Design review of the part built by this model. Coordinates are the model's own, in mm. Coordinates: 2 decimals unless noted, no trailing zeros. Loops run counter-clockwise (first coordinate to the right, second up) from the corner with the lowest first, then second, coordinate; pieces in that order, holes last. Notation, with made-up numbers: (-9, 27) -> (0, 27) arc R18 cw to (0, 32) -> close; hole circle Ø4 at (-35.5, 41). An arc over 180 degrees is marked (long way). Use one line per item in the form item = value. Start each with the question number.
1. Consider section A-A (z = 17.5). State the section outline as (x, y) points, then the cut area to 3 significant figures.
2. Consider section B-B (x = -33). State the section outline as (y, z) points.
3. For pin 1 (1.3 mm diameter, centred on y = 1, z = -22.5, fed in from -X); pin 2 (1.3 mm diameter, centred on y = 1.5, z = 18, fed in from +X), all flat-tipped, find the tip position at first contact; note any pin that passes through.
4. Wall thickness on line 1 (X direction, y = 0.9, z = 3.5); line 2 (Z direction, x = 44, y = 1.55): over which ranges is each line inside the solid? List them lowest first. Write a range as from..to.
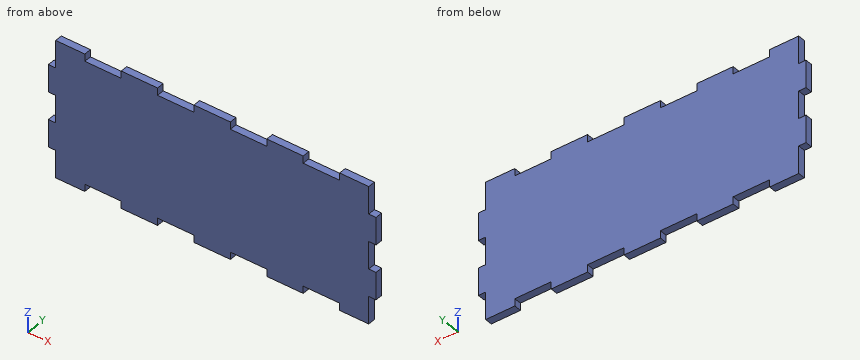
from build123d import *

# Parameters (mm, degrees)
SKETCH1_W           = 114.3
SKETCH1_H           = 48.006
BOSS_EXTRUDE1_DEPTH = 2.54
CUT_EXTRUDE2_REACH  = 64.038
SKETCH2_W           = 2.54
SKETCH2_H           = 9.6012
SKETCH2_W_2         = 12.7
SKETCH2_H_2         = 2.54


with BuildPart() as part:
    # Sketch1 → Boss-Extrude1 (new body)
    with BuildSketch(Plane(origin=(0, 0, 0), x_dir=(1, 0, 0), z_dir=(0, 1, 0))):
        Rectangle(SKETCH1_W, SKETCH1_H)
    extrude(amount=BOSS_EXTRUDE1_DEPTH)

    # Sketch2 → Cut-Extrude2 (cut, up to next)
    with BuildSketch(Plane(origin=(0, 2.54, 0), x_dir=(1, 0, 0), z_dir=(0, 1, 0)), mode=Mode.PRIVATE) as cut_extrude2_sk1:
        with Locations((-55.88, 19.2024)):
            Rectangle(SKETCH2_W, SKETCH2_H)
    cut_extrude2_tool1 = extrude(cut_extrude2_sk1.sketch, amount=-CUT_EXTRUDE2_REACH, mode=Mode.PRIVATE) & part.part
    # Sketch2 → Cut-Extrude2 (cut, up to next)
    with BuildSketch(Plane(origin=(0, 2.54, 0), x_dir=(1, 0, 0), z_dir=(0, 1, 0)), mode=Mode.PRIVATE) as cut_extrude2_sk2:
        with Locations((-38.1, 22.733)):
            Rectangle(SKETCH2_W_2, SKETCH2_H_2)
    cut_extrude2_tool2 = extrude(cut_extrude2_sk2.sketch, amount=-CUT_EXTRUDE2_REACH, mode=Mode.PRIVATE) & part.part
    # Sketch2 → Cut-Extrude2 (cut, up to next)
    with BuildSketch(Plane(origin=(0, 2.54, 0), x_dir=(1, 0, 0), z_dir=(0, 1, 0)), mode=Mode.PRIVATE) as cut_extrude2_sk3:
        with Locations((-12.7, 22.733)):
            Rectangle(SKETCH2_W_2, SKETCH2_H_2)
    cut_extrude2_tool3 = extrude(cut_extrude2_sk3.sketch, amount=-CUT_EXTRUDE2_REACH, mode=Mode.PRIVATE) & part.part
    # Sketch2 → Cut-Extrude2 (cut, up to next)
    with BuildSketch(Plane(origin=(0, 2.54, 0), x_dir=(1, 0, 0), z_dir=(0, 1, 0)), mode=Mode.PRIVATE) as cut_extrude2_sk4:
        with Locations((12.7, 22.733)):
            Rectangle(SKETCH2_W_2, SKETCH2_H_2)
    cut_extrude2_tool4 = extrude(cut_extrude2_sk4.sketch, amount=-CUT_EXTRUDE2_REACH, mode=Mode.PRIVATE) & part.part
    # Sketch2 → Cut-Extrude2 (cut, up to next)
    with BuildSketch(Plane(origin=(0, 2.54, 0), x_dir=(1, 0, 0), z_dir=(0, 1, 0)), mode=Mode.PRIVATE) as cut_extrude2_sk5:
        with Locations((38.1, 22.733)):
            Rectangle(SKETCH2_W_2, SKETCH2_H_2)
    cut_extrude2_tool5 = extrude(cut_extrude2_sk5.sketch, amount=-CUT_EXTRUDE2_REACH, mode=Mode.PRIVATE) & part.part
    # Sketch2 → Cut-Extrude2 (cut, up to next)
    with BuildSketch(Plane(origin=(0, 2.54, 0), x_dir=(1, 0, 0), z_dir=(0, 1, 0)), mode=Mode.PRIVATE) as cut_extrude2_sk6:
        with Locations((55.88, 19.2024)):
            Rectangle(SKETCH2_W, SKETCH2_H)
    cut_extrude2_tool6 = extrude(cut_extrude2_sk6.sketch, amount=-CUT_EXTRUDE2_REACH, mode=Mode.PRIVATE) & part.part
    # Sketch2 → Cut-Extrude2 (cut, up to next)
    with BuildSketch(Plane(origin=(0, 2.54, 0), x_dir=(1, 0, 0), z_dir=(0, 1, 0)), mode=Mode.PRIVATE) as cut_extrude2_sk7:
        with Locations((55.88, 0)):
            Rectangle(SKETCH2_W, SKETCH2_H)
    cut_extrude2_tool7 = extrude(cut_extrude2_sk7.sketch, amount=-CUT_EXTRUDE2_REACH, mode=Mode.PRIVATE) & part.part
    # Sketch2 → Cut-Extrude2 (cut, up to next)
    with BuildSketch(Plane(origin=(0, 2.54, 0), x_dir=(1, 0, 0), z_dir=(0, 1, 0)), mode=Mode.PRIVATE) as cut_extrude2_sk8:
        with Locations((55.88, -19.2024)):
            Rectangle(SKETCH2_W, SKETCH2_H)
    cut_extrude2_tool8 = extrude(cut_extrude2_sk8.sketch, amount=-CUT_EXTRUDE2_REACH, mode=Mode.PRIVATE) & part.part
    # Sketch2 → Cut-Extrude2 (cut, up to next)
    with BuildSketch(Plane(origin=(0, 2.54, 0), x_dir=(1, 0, 0), z_dir=(0, 1, 0)), mode=Mode.PRIVATE) as cut_extrude2_sk9:
        with Locations((38.1, -22.733)):
            Rectangle(SKETCH2_W_2, SKETCH2_H_2)
    cut_extrude2_tool9 = extrude(cut_extrude2_sk9.sketch, amount=-CUT_EXTRUDE2_REACH, mode=Mode.PRIVATE) & part.part
    # Sketch2 → Cut-Extrude2 (cut, up to next)
    with BuildSketch(Plane(origin=(0, 2.54, 0), x_dir=(1, 0, 0), z_dir=(0, 1, 0)), mode=Mode.PRIVATE) as cut_extrude2_sk10:
        with Locations((12.7, -22.733)):
            Rectangle(SKETCH2_W_2, SKETCH2_H_2)
    cut_extrude2_tool10 = extrude(cut_extrude2_sk10.sketch, amount=-CUT_EXTRUDE2_REACH, mode=Mode.PRIVATE) & part.part
    # Sketch2 → Cut-Extrude2 (cut, up to next)
    with BuildSketch(Plane(origin=(0, 2.54, 0), x_dir=(1, 0, 0), z_dir=(0, 1, 0)), mode=Mode.PRIVATE) as cut_extrude2_sk11:
        with Locations((-12.7, -22.733)):
            Rectangle(SKETCH2_W_2, SKETCH2_H_2)
    cut_extrude2_tool11 = extrude(cut_extrude2_sk11.sketch, amount=-CUT_EXTRUDE2_REACH, mode=Mode.PRIVATE) & part.part
    # Sketch2 → Cut-Extrude2 (cut, up to next)
    with BuildSketch(Plane(origin=(0, 2.54, 0), x_dir=(1, 0, 0), z_dir=(0, 1, 0)), mode=Mode.PRIVATE) as cut_extrude2_sk12:
        with Locations((-38.1, -22.733)):
            Rectangle(SKETCH2_W_2, SKETCH2_H_2)
    cut_extrude2_tool12 = extrude(cut_extrude2_sk12.sketch, amount=-CUT_EXTRUDE2_REACH, mode=Mode.PRIVATE) & part.part
    # Sketch2 → Cut-Extrude2 (cut, up to next)
    with BuildSketch(Plane(origin=(0, 2.54, 0), x_dir=(1, 0, 0), z_dir=(0, 1, 0)), mode=Mode.PRIVATE) as cut_extrude2_sk13:
        with Locations((-55.88, -19.2024)):
            Rectangle(SKETCH2_W, SKETCH2_H)
    cut_extrude2_tool13 = extrude(cut_extrude2_sk13.sketch, amount=-CUT_EXTRUDE2_REACH, mode=Mode.PRIVATE) & part.part
    # Sketch2 → Cut-Extrude2 (cut, up to next)
    with BuildSketch(Plane(origin=(0, 2.54, 0), x_dir=(1, 0, 0), z_dir=(0, 1, 0)), mode=Mode.PRIVATE) as cut_extrude2_sk14:
        with Locations((-55.88, 0)):
            Rectangle(SKETCH2_W, SKETCH2_H)
    cut_extrude2_tool14 = extrude(cut_extrude2_sk14.sketch, amount=-CUT_EXTRUDE2_REACH, mode=Mode.PRIVATE) & part.part
    add(cut_extrude2_tool1.solids().sort_by_distance((-55.88, 2.54, -19.2024))[0], mode=Mode.SUBTRACT)
    add(cut_extrude2_tool2.solids().sort_by_distance((-38.1, 2.54, -22.733))[0], mode=Mode.SUBTRACT)
    add(cut_extrude2_tool3.solids().sort_by_distance((-12.7, 2.54, -22.733))[0], mode=Mode.SUBTRACT)
    add(cut_extrude2_tool4.solids().sort_by_distance((12.7, 2.54, -22.733))[0], mode=Mode.SUBTRACT)
    add(cut_extrude2_tool5.solids().sort_by_distance((38.1, 2.54, -22.733))[0], mode=Mode.SUBTRACT)
    add(cut_extrude2_tool6.solids().sort_by_distance((55.88, 2.54, -19.2024))[0], mode=Mode.SUBTRACT)
    add(cut_extrude2_tool7.solids().sort_by_distance((55.88, 2.54, 0))[0], mode=Mode.SUBTRACT)
    add(cut_extrude2_tool8.solids().sort_by_distance((55.88, 2.54, 19.2024))[0], mode=Mode.SUBTRACT)
    add(cut_extrude2_tool9.solids().sort_by_distance((38.1, 2.54, 22.733))[0], mode=Mode.SUBTRACT)
    add(cut_extrude2_tool10.solids().sort_by_distance((12.7, 2.54, 22.733))[0], mode=Mode.SUBTRACT)
    add(cut_extrude2_tool11.solids().sort_by_distance((-12.7, 2.54, 22.733))[0], mode=Mode.SUBTRACT)
    add(cut_extrude2_tool12.solids().sort_by_distance((-38.1, 2.54, 22.733))[0], mode=Mode.SUBTRACT)
    add(cut_extrude2_tool13.solids().sort_by_distance((-55.88, 2.54, 19.2024))[0], mode=Mode.SUBTRACT)
    add(cut_extrude2_tool14.solids().sort_by_distance((-55.88, 2.54, 0))[0], mode=Mode.SUBTRACT)


solid = part.part
Geometry check:
q1.outline = (-54.61, 0) -> (54.61, 0) -> (54.61, 2.54) -> (-54.61, 2.54) -> close
q1.area = 277 mm²
q2.outline = (0, -21.46) -> (2.54, -21.46) -> (2.54, 21.46) -> (0, 21.46) -> close
q3.pin_1 = -54.61
q3.pin_2 = 54.61
q4.line_1 = -54.61..54.61
q4.line_2 = -21.46..21.46
